The model under review builds one solid part; all positions refer to its coordinate system, in mm. Face numbers are marked on the shaded views. Coordinates: 2 decimals unless noted, no trailing zeros. Loops run counter-clockwise (first coordinate to the right, second up) from the corner with the lowest first, then second, coordinate; pieces in that order, holes last. Notation, with made-up numbers: M -27.5,88 L 27.5,88 A20 cw 27.5,125 Z; hole C 60.25,53.25 d5. An arc over 180 degrees is marked long. Return JSON: item names as keys, results as strings.
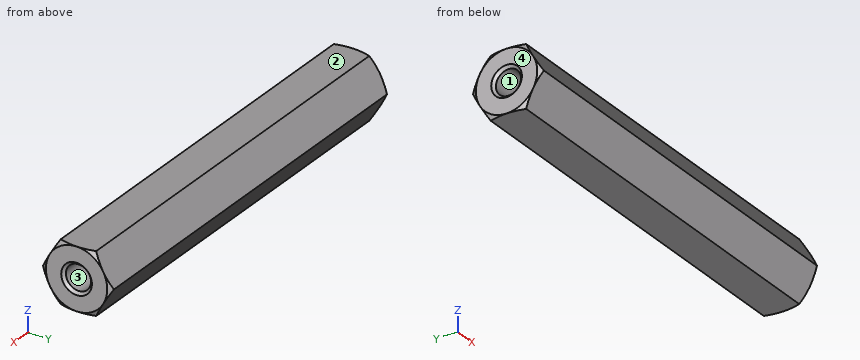
Autodesk Inventor part; units mm, degrees
ref_plane "C3_XY" through (39.5, 0, 0) normal (-1, 0, 0) x (0, 0, -1)
ref_plane "C3_YZ" through (39.5, 0, 0) normal (0, 0, -1) x (0, -1, 0)
ref_plane "C3_ZX" through (39.5, 0, 0) normal (0, -1, 0) x (-1, 0, 0)
sketch "Sketch_1" plane through (0, 0, 0) normal (0, 0, 1) x (1, 0, 0)
  line L0 (39.5, 0) -> (0, 0)
  line L1 (0, 0) -> (0, 3)
  line L2 (0, 3) -> (0.5485, 3.95)
  line L3 (0.5485, 3.95) -> (38.9515, 3.95)
  line L4 (38.9515, 3.95) -> (39.5, 3)
  line L5 (39.5, 3) -> (39.5, 0)
  line L6 (39.5, 0) -> (0, 0)
revolve "Revolution1" add sketch "Sketch_1" angle 360 about axis through (39.5, 0, 0) along (1, 0, 0)
sketch "Sketch_2" plane through (0, 0, 0) normal (1, 0, 0) x (0, 1, 0)
  line L0 (6, 6) -> (-6, 6)
  line L1 (-6, 6) -> (-6, -6)
  line L2 (-6, -6) -> (6, -6)
  line L3 (6, -6) -> (6, 6)
  line L4 (-1.7321, 3) -> (-3.4641, 0)
  line L5 (-3.4641, 0) -> (-1.7321, -3)
  line L6 (-1.7321, -3) -> (1.7321, -3)
  line L7 (1.7321, -3) -> (3.4641, 0)
  line L8 (3.4641, 0) -> (1.7321, 3)
  line L9 (1.7321, 3) -> (-1.7321, 3)
extrude "Extrusion1" cut sketch "Sketch_2" along normal blind 39.5
sketch "Sketch3" plane through (0, 0, 0) normal (-1, 0, 0) x (0, 0, 1)
  point P0 (0, 0)
hole "Hole1" at (0, 0, 0) direction (1, 0, 0) diameter 2.459 depth 8.2901 tip angle 120 countersink diameter 3 countersink angle 90
sketch "Sketch4" plane through (39.5, 0, 0) normal (1, 0, 0) x (0, 0, -1)
  point P0 (0, 0)
hole "Hole2" at (39.5, 0, 0) direction (-1, 0, 0) diameter 2.459 depth 8.2901 tip angle 120 countersink diameter 3 countersink angle 90
ref_plane "C3_XY" through (39.5, 0, 0) normal (-1, 0, 0) x (0, 0, -1)
ref_plane "C3_YZ" through (39.5, 0, 0) normal (0, 0, -1) x (0, -1, 0)
ref_plane "C3_ZX" through (39.5, 0, 0) normal (0, -1, 0) x (-1, 0, 0)
properties part number "ABLSBF6-39.5-M3-N3" material "Aluminum 2014-T4"
1. To check wall thickness, follow line 1 (Z direction, x = 34.5, y = 0); line 2 (Y direction, x = 6, z = -0.6); line 3 (Z direction, x = 19.5, y = 3). State the ranges of each line that lie inside material, in increasing order.
Check values:
{"line 1": "-3 to -1.23, 1.23 to 3", "line 2": "-3.12 to -1.07, 1.07 to 3.12", "line 3": "-0.8 to 0.8"}
2. The part is to be moulded in two halves that separate along Z. For the marked faces 1, 2, 3 and 4, say which applies: released by +Z, released by -Z, zero draft, split by the parting line, or undercut.
Check values:
{"face 1": "undercut", "face 2": "released by +Z", "face 3": "undercut", "face 4": "zero draft"}
3. Add section B-B on x = 23. Give the boundary of the cut face in (y, z), plus the area to 3 significant figures.
Check values:
{"outline": "M -3.46,0 L -1.73,-3 L 1.73,-3 L 3.46,0 L 1.73,3 L -1.73,3 Z", "area": "31.2 mm²"}
4. Insertion check: pin 1 Ø1.5 at (y, z) = (0, 0) entering from +X. The pin has a flat end and moves straight along its axis. Give the tip position at first contact, or say it passes through.
Check values:
{"pin 1": "x = 30.93"}
5. Add section A-A on x = 32. Give the boundary of the cut face in (y, z).
Check values:
{"outline": "M -3.46,0 L -1.73,-3 L 1.73,-3 L 3.46,0 L 1.73,3 L -1.73,3 Z; hole C 0,0 d2.46"}
